For this review, take the finished solid that the model builds, in its own axes (mm). Face numbers are marked on the shaded views. Coordinates: 2 decimals unless noted, no trailing zeros. Write each loop counter-clockwise with the first axis right and the second up, starting at its lowest first coordinate (ties: lowest second). Pieces come first, ordered by that corner, then holes. Notation, with made-up numbers: M 28,74.5 L 47,74.5 A10 cw 47,93.5 Z; hole C 60,66 d11. An arc over 180 degrees is marked long. One line per question, with ' | ' between items.
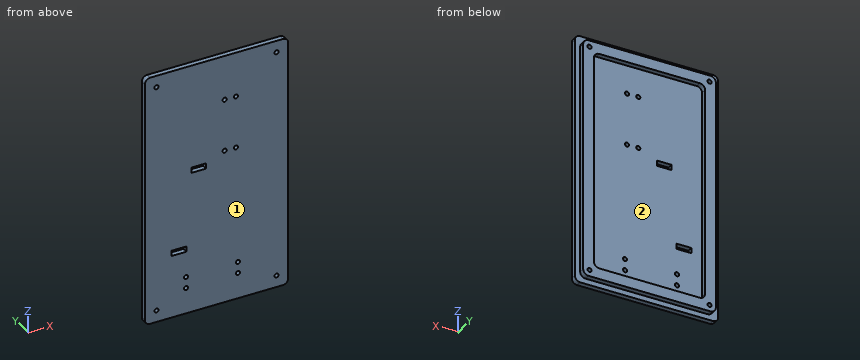
from build123d import *

# Parameters (mm, degrees)
BOSS_EXTRUDE1_DEPTH = 3
BOSS_EXTRUDE2_DEPTH = 3
SKETCH3_R           = 1.15
CUT_EXTRUDE1_DEPTH  = 162.356747612
SKETCH4_W           = 8.2
SKETCH4_H           = 3
CUT_EXTRUDE2_DEPTH  = 10
SKETCH5_R           = 1.15
CUT_EXTRUDE3_DEPTH  = 3
SKETCH6_R           = 1.15
CUT_EXTRUDE4_DEPTH  = 3


with BuildPart() as part:
    # Sketch1 → Boss-Extrude1 (new body)
    with BuildSketch(Plane(origin=(0, 0, 0), x_dir=(1, 0, 0), z_dir=(0, 1, 0))):
        with BuildLine():
            Line((3, 0), (77, 0))
            ThreePointArc((77, 0), (79.121320344, 0.878679656), (80, 3))
            Line((80, 3), (80, 137))
            ThreePointArc((80, 137), (79.121320344, 139.121320344), (77, 140))
            Line((77, 140), (3, 140))
            ThreePointArc((3, 140), (0.878679656, 139.121320344), (0, 137))
            Line((0, 137), (0, 3))
            ThreePointArc((0, 3), (0.878679656, 0.878679656), (3, 0))
        make_face()
    extrude(amount=BOSS_EXTRUDE1_DEPTH)

    # Sketch2 → Boss-Extrude2 (add)
    with BuildSketch(Plane(origin=(0, 3, 0), x_dir=(1, 0, 0), z_dir=(0, 1, 0))):
        with BuildLine():
            Line((6, 137), (74, 137))
            ThreePointArc((74, 137), (76.121320344, 136.121320344), (77, 134))
            Line((77, 134), (77, 6))
            ThreePointArc((77, 6), (76.121320344, 3.878679656), (74, 3))
            Line((74, 3), (6, 3))
            ThreePointArc((6, 3), (3.878679656, 3.878679656), (3, 6))
            Line((3, 6), (3, 134))
            ThreePointArc((3, 134), (3.878679656, 136.121320344), (6, 137))
        make_face()
        with BuildLine():
            Line((12, 131), (68, 131))
            ThreePointArc((68, 131), (70.121320344, 130.121320344), (71, 128))
            Line((71, 128), (71, 12))
            ThreePointArc((71, 12), (70.121320344, 9.878679656), (68, 9))
            Line((68, 9), (12, 9))
            ThreePointArc((12, 9), (9.878679656, 9.878679656), (9, 12))
            Line((9, 12), (9, 128))
            ThreePointArc((9, 128), (9.878679656, 130.121320344), (12, 131))
        make_face(mode=Mode.SUBTRACT)
    extrude(amount=BOSS_EXTRUDE2_DEPTH)

    # Sketch3 → Cut-Extrude1 (cut, through all)
    with BuildSketch(Plane(origin=(0, 6, 0), x_dir=(1, 0, 0), z_dir=(0, 1, 0))):
        with Locations(Location((6.5, 133.5, 0), (0, 0, 270))):
            Circle(SKETCH3_R)
        with Locations(Location((73.5, 133.5, 0), (0, 0, 270))):
            Circle(SKETCH3_R)
        with Locations(Location((73.5, 6.5, 0), (0, 0, 270))):
            Circle(SKETCH3_R)
        with Locations(Location((6.5, 6.5, 0), (0, 0, 270))):
            Circle(SKETCH3_R)
    extrude(amount=-CUT_EXTRUDE1_DEPTH, mode=Mode.SUBTRACT)

    # Sketch4 → Cut-Extrude2 (cut)
    with BuildSketch(Plane.XZ):
        with Locations((30.1, -59.5)):
            Rectangle(SKETCH4_W, SKETCH4_H)
        with Locations((19.1, -103.5)):
            Rectangle(SKETCH4_W, SKETCH4_H)
    extrude(amount=-CUT_EXTRUDE2_DEPTH, mode=Mode.SUBTRACT)

    # Sketch5 → Cut-Extrude3 (cut)
    with BuildSketch(Plane.XZ):
        with Locations(Location((23, -125.65, 0), (0, 0, 270))):
            Circle(SKETCH5_R)
        with Locations(Location((52, -125.65, 0), (0, 0, 270))):
            Circle(SKETCH5_R)
        with Locations(Location((52, -119.35, 0), (0, 0, 270))):
            Circle(SKETCH5_R)
        with Locations(Location((23, -119.35, 0), (0, 0, 270))):
            Circle(SKETCH5_R)
    extrude(amount=-CUT_EXTRUDE3_DEPTH, mode=Mode.SUBTRACT)

    # Sketch6 → Cut-Extrude4 (cut)
    with BuildSketch(Plane.XZ):
        with Locations(Location((50.88, -53.92, 0), (0, 0, 270))):
            Circle(SKETCH6_R)
        with Locations(Location((44.58, -53.92, 0), (0, 0, 270))):
            Circle(SKETCH6_R)
        with Locations(Location((50.88, -24.92, 0), (0, 0, 270))):
            Circle(SKETCH6_R)
        with Locations(Location((44.58, -24.92, 0), (0, 0, 270))):
            Circle(SKETCH6_R)
    extrude(amount=-CUT_EXTRUDE4_DEPTH, mode=Mode.SUBTRACT)


solid = part.part
1) Insertion check: pin 1 Ø12 at (x, z) = (41, -112.5) entering from +Y; pin 2 Ø0.9 at (x, y) = (56.5, 4) entering from +Z; pin 3 Ø0.9 at (y, z) = (4.5, -58) entering from -X. Each pin has a flat end and moves straight along its axis. Give the tip position at first contact, or say it passes through.
Responses:
pin 1: y = 3 | pin 2: z = -3 | pin 3: x = 3
2) We need section A-A on z = -72.5. State the section outline as (x, y) points.
Responses:
outline: M 0,0 L 80,0 L 80,3 L 77,3 L 77,6 L 71,6 L 71,3 L 9,3 L 9,6 L 3,6 L 3,3 L 0,3 Z
3) To check wall thickness, follow line 1 along Z through (x, y) = (73.5, 1.85); line 2 along X through (y, z) = (2.1, -24.92); line 3 along X through (y, z) = (1.5, -119.35). State the ranges of each line that lie inside material, in increasing order. Write a range as [from, to].
Responses:
line 1: [-140, -134.65], [-132.35, -7.65], [-5.35, 0] | line 2: [0, 43.43], [45.73, 49.73], [52.03, 80] | line 3: [0, 21.85], [24.15, 50.85], [53.15, 80]
4) The part is to be moulded in two halves that separate along Z. For the marked faces 1 and 2, say which applies: +Z half, -Z half, draft (parallel to the pull), parting line (faces both ways), or undercut.
Responses:
face 1: draft | face 2: undercut
